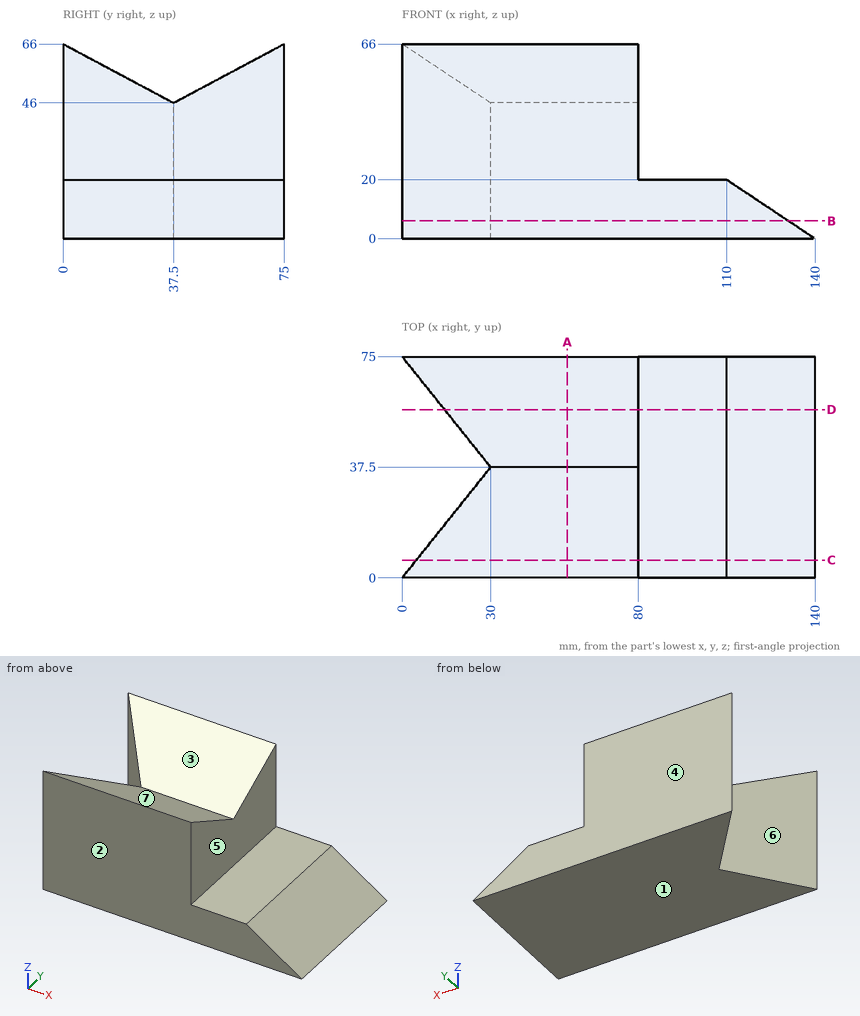
Job drawing, mm, ordinate dimensions from the low corner. One solid piece. A direction names the side the tool comes from. Round coordinates to 2 decimals unless told otherwise and drop trailing zeros. Loops run counter-clockwise (first coordinate to the right, second up) from the corner with the lowest first, then second, coordinate; pieces in that order, holes last. Notation, with made-up numbers: (40, 82) -> (63, 82) arc R21 cw to (63, 112) -> close; hole circle Ø7 at (77.5, 57). An arc over 180 degrees is marked (long way). Use a Markdown table: item, result.
1) Tool access for the marked faces 5, 6 and 7: list every direction of +Z, -Z, +X, -X, +Y, -Y with a clear straight run to the whole face (end or side of a thin tool).
The answers:
| item | result |
|---|---|
| face 5 | +Z, +X, +Y, -Y |
| face 6 | +Z, -Z, -X |
| face 7 | +Z, +X, -X |
2) Cut at A-A, the plane x = 56. List the corners of the cut face in (y, z), and give its area (3 significant figures).
The answers:
| item | result |
|---|---|
| outline | (0, 0) -> (75, 0) -> (75, 66) -> (37.5, 46) -> (0, 66) -> close |
| area | 4,200 mm2 |
3) Pull direction Y, two halves, no side cores. Call the marked faces 1, 2, 3 and 4: pulls with the +Y half, pulls with the -Y half, needs draft (parallel to the pull), parting line crosses it, or undercut.
The answers:
| item | result |
|---|---|
| face 1 | needs draft |
| face 2 | pulls with the -Y half |
| face 3 | undercut |
| face 4 | pulls with the +Y half |
4) Probe line 1 (Y direction, x = 17, z = 28); line 2 (Z direction, x = 83, y = 44.5); line 3 (Y direction, x = 19, z = 32). List the from-to ranges inside material, lowest first. Write a range as [from, to].
The answers:
| item | result |
|---|---|
| line 1 | y = [0, 21.25], [53.75, 75] |
| line 2 | z = [0, 20] |
| line 3 | y = [0, 23.75], [51.25, 75] |
5) Cut at C-C, the plane y = 6. List the corners of the cut face in (x, z).
The answers:
| item | result |
|---|---|
| outline | (4.8, 0) -> (140, 0) -> (110, 20) -> (80, 20) -> (80, 62.8) -> (4.8, 62.8) -> close |
6) Drop flat-ended pins along their axis: pin 1 Ø23 at (y, z) = (45.5, 51.5) entering from +X; pin 2 Ø15 at (x, y) = (88, 31) entering from +Z. Give the stop position or say it passes through.
The answers:
| item | result |
|---|---|
| pin 1 | stops at x = 80 |
| pin 2 | stops at z = 20 |
7) Cut at D-D, the plane y = 57. List the corners of the cut face in (x, z).
The answers:
| item | result |
|---|---|
| outline | (14.4, 0) -> (140, 0) -> (110, 20) -> (80, 20) -> (80, 56.4) -> (14.4, 56.4) -> close |
8) Cut at B-B, the plane z = 6. List the corners of the cut face in (x, y), and give its area (3 significant figures).
The answers:
| item | result |
|---|---|
| outline | (0, 0) -> (131, 0) -> (131, 75) -> (0, 75) -> (30, 37.5) -> close |
| area | 8,700 mm2 |
